Source: three-view drawing plus pictorial views. Frame: mm from the lowest corner of the part. Give positions to 0.01 mm unless a question says otherwise; leave off trailing zeros. Order: outer loops, then holes, each group sorted by start corner. A loop starts at its lowest first (then second) coordinate and runs counter-clockwise, first axis right, second up.
1) First-contact query: P1, Ø2.5, axis at x = 35, z = 4.5, coming from the +Y side; P2, Ø8, axis at x = 51, z = 16, coming from the +Y side; P3, Ø1.5, axis at y = 47, z = 4, coming from the +X side. Flat tips, straight axial feed; report the tip coordinate or a pass-through.
2) Section A-A, the plane z = 4.75. Return loops of the section in (x, y), plus the area to 3 significant figures.
3) Section C-C, the plane x = 33. Return loops of the section in (y, z), plus the area to 3 significant figures.
4) Material intervals for line 1 (Y direction, x = 33, z = 6.75); line 2 (Y direction, x = 33, z = 7.75); line 3 (X direction, y = 44, z = 4.25), sorted ascending.
5) Section D-D, the plane y = 11. Return loops of the section in (x, z), plus the area to 3 significant figures.
6) Section B-B, the plane y = 33. Return loops of the section in (x, z).
7) Draft query along X for the marked faces 1, 2 and 3. Return one class per face: released by +X, released by -X, zero draft, split by the parting line, or undercut.
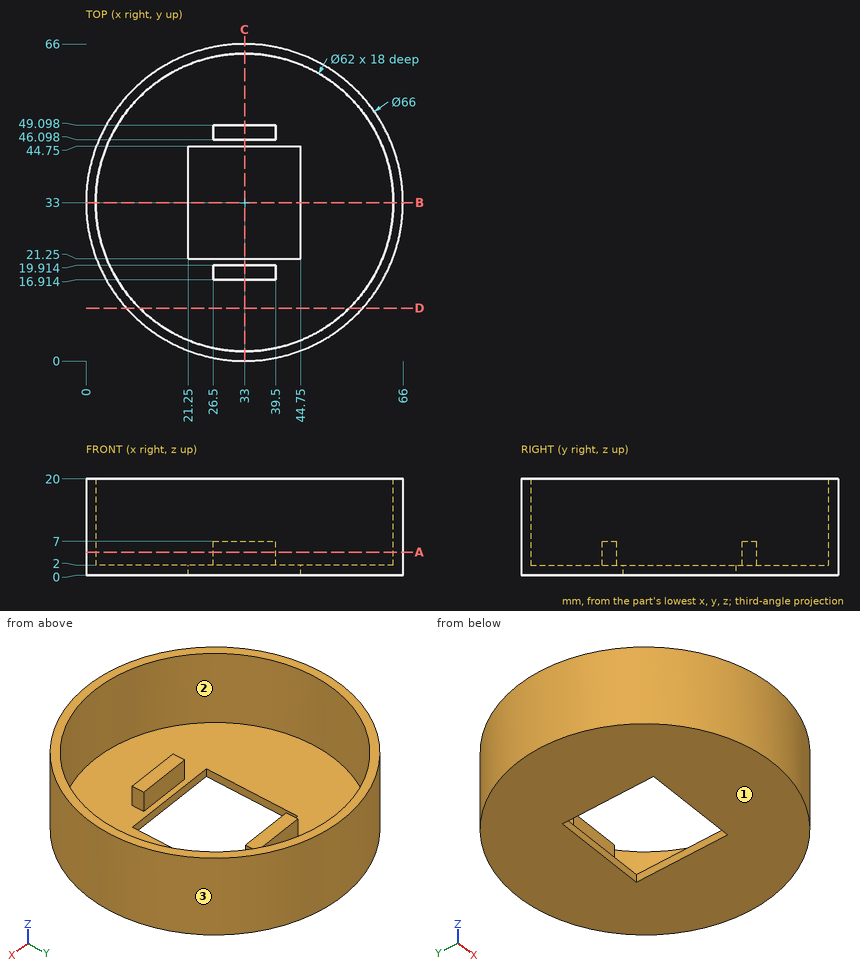
From the geometry:
1. P1: stops at y = 65.99
1. P2: stops at y = 62.88
1. P3: stops at x = 63.22
2. outline: circle Ø66 at (33, 33); (26.5, 16.91) - (39.5, 16.91) - (39.5, 19.91) - (26.5, 19.91) - close; (26.5, 46.1) - (39.5, 46.1) - (39.5, 49.1) - (26.5, 49.1) - close; hole circle Ø62 at (33, 33)
2. area: 480 mm2
3. outline: (0, 0) - (21.25, 0) - (21.25, 2) - (19.91, 2) - (19.91, 7) - (16.91, 7) - (16.91, 2) - (2, 2) - (2, 20) - (0, 20) - close; (44.75, 0) - (66, 0) - (66, 20) - (64, 20) - (64, 2) - (49.1, 2) - (49.1, 7) - (46.1, 7) - (46.1, 2) - (44.75, 2) - close
3. area: 187 mm2
4. line 1: y = 0 to 2, 16.91 to 19.91, 46.1 to 49.1, 64 to 66
4. line 2: y = 0 to 2, 64 to 66
4. line 3: x = 1.89 to 4.02, 61.98 to 64.11
5. outline: (8.4, 0) - (57.6, 0) - (57.6, 20) - (54.84, 20) - (54.84, 2) - (11.16, 2) - (11.16, 20) - (8.4, 20) - close
5. area: 198 mm2
6. outline: (0, 0) - (21.25, 0) - (21.25, 2) - (2, 2) - (2, 20) - (0, 20) - close; (44.75, 0) - (66, 0) - (66, 20) - (64, 20) - (64, 2) - (44.75, 2) - close
7. face 1: zero draft
7. face 2: undercut
7. face 3: split by the parting line
